Verification items for the finished model (mm, model axes). A direction names the side the tool comes from. Round coordinates to 2 decimals unless told otherwise and drop trailing zeros. Write each loop counter-clockwise with the first axis right and the second up, starting at its lowest first coordinate (ties: lowest second). Pieces come first, ordered by that corner, then holes. Notation, with made-up numbers: (-20.75, -30.75) -> (11.25, -30.75) arc R8 ccw to (11.25, -19.75) -> close; hole circle Ø6 at (39.25, 74). An arc over 180 degrees is marked (long way). Answer as a JSON object with one key per item and string values. Group by question number.
(1) Sectioned sample at B-B on z = 25.5. Record the cut outline in (x, y) (3 decimals).
(2) Sectioned sample at A-A on x = 57. Record the cut outline in (y, z) (3 decimals), and give its area (3 significant figures).
(3) Sectioned sample at C-C on z = -37.5. Record the cut outline in (x, y) (3 decimals).
(4) Sectioned sample at D-D on z = 15. Record the cut outline in (x, y) (3 decimals), and give its area (3 significant figures).
(5) Set-up check for faces 4 (the face through (-4, 20.955, -31)), 5 (the face through (-79.106, 21.878, 0.284)), 6 (the face through (89, 22.225, 1)), 7 (the face through (89, 13, -41.275)), 8 (the face through (5, 22.225, -29)): record each of +Z, -Z, +X, -X, +Y, -Y from which the full face is reachable in a straight line by a thin tool's end or side.
(6) Scan lines: L1, parallel to X at y = 15.5, z = -22 (3 decimals); L2, parallel to Z at x = -49, y = 14.5 (3 decimals); L3, parallel to X at y = 23, z = -12 (3 decimals). Record each from-to range of solid material in increasing order. Write a range as from..to.
(7) Draft check along X on faces 1 (the face through (66.675, 9, 14)), 2 (the face through (-82.55, 7, 1)), 3 (the face through (81, 16, -6.35)). Enter one of: released by +X, released by -X, zero draft, split by the parting line, or undercut.
(8) Gauge pin test, flat ends, axial feed: pin 1 Ø3 at (y, z) = (15, 8) entering from -X (3 decimals); pin 2 Ø1 at (x, z) = (24.5, 28.5) entering from +Y (3 decimals); pin 3 Ø0.7 at (x, z) = (78.5, -6.5) entering from -Y (3 decimals). Record the tip position at first contact, or that the pin passes through.
```python
from build123d import *

# Parameters (mm, degrees)
SKETCH1_W           = 165.1
SKETCH1_H           = 88.9
BOSS_EXTRUDE1_DEPTH = 25.4
SKETCH2_W           = 82.55
SKETCH2_H           = 19.05
BOSS_EXTRUDE2_DEPTH = 12.7
SKETCH5_W           = 151.13
SKETCH5_H           = 70.358
CUT_EXTRUDE3_DEPTH  = 3.175
SKETCH7_W           = 165.1
SKETCH7_H           = 88.9
CUT_EXTRUDE4_DEPTH  = 3.175
CUT_EXTRUDE5_DEPTH  = 29.21
SKETCH11_W          = 142.477455076
SKETCH11_H          = 82.55
CUT_EXTRUDE7_DEPTH  = 17.78
SKETCH15_W          = 137.668
SKETCH15_H          = 57.404
CUT_EXTRUDE8_DEPTH  = 6.35
SKETCH19_W          = 12.7
SKETCH19_H          = 24.13
CUT_EXTRUDE9_DEPTH  = 17.78
SKETCH22_W          = 19.304
SKETCH22_H          = 12.7
CUT_EXTRUDE11_DEPTH = 7.62
CUT_EXTRUDE11_DRAFT = 15
SKETCH24_W          = 28.575
SKETCH24_H          = 19.05
CUT_EXTRUDE12_DEPTH = 5.08
CUT_EXTRUDE14_DEPTH = 30.48


with BuildPart() as part:
    # Sketch1 → Boss-Extrude1 (new body)
    with BuildSketch(Plane(origin=(0, 0, 0), x_dir=(1, 0, 0), z_dir=(0, 1, 0))):
        Rectangle(SKETCH1_W, SKETCH1_H)
    extrude(amount=BOSS_EXTRUDE1_DEPTH)

    # Sketch2 → Boss-Extrude2 (add)
    with BuildSketch(Plane(origin=(82.55, 0, 0), x_dir=(0, 0, -1), z_dir=(1, 0, 0))):
        with Locations((0, 12.7)):
            Rectangle(SKETCH2_W, SKETCH2_H)
    extrude(amount=BOSS_EXTRUDE2_DEPTH)

    # Sketch5 → Cut-Extrude3 (cut)
    with BuildSketch(Plane(origin=(0, 25.4, 0), x_dir=(1, 0, 0), z_dir=(0, 1, 0))):
        Rectangle(SKETCH5_W, SKETCH5_H)
    extrude(amount=-CUT_EXTRUDE3_DEPTH, mode=Mode.SUBTRACT)

    # Sketch7 → Cut-Extrude4 (cut)
    with BuildSketch(Plane.XZ):
        Rectangle(SKETCH7_W, SKETCH7_H)
    extrude(amount=-CUT_EXTRUDE4_DEPTH, mode=Mode.SUBTRACT)

    # Sketch9 → Cut-Extrude5 (cut)
    with BuildSketch(Plane(origin=(95.25, 0, 0), x_dir=(0, 0, -1), z_dir=(1, 0, 0))):
        with BuildLine():
            Line((6.985, 4.445), (-6.985, 4.445))
            ThreePointArc((-6.985, 4.445), (-12.065, 9.525), (-6.985, 14.605))
            Line((-6.985, 14.605), (6.985, 14.605))
            ThreePointArc((6.985, 14.605), (12.065, 9.525), (6.985, 4.445))
        make_face()
    extrude(amount=-CUT_EXTRUDE5_DEPTH, mode=Mode.SUBTRACT)

    # Sketch11 → Cut-Extrude7 (cut)
    with BuildSketch(Plane(origin=(0, 3.175, 0), x_dir=(-1, 0, 0), z_dir=(0, -1, 0))):
        with Locations((4.563727538, 0)):
            Rectangle(SKETCH11_W, SKETCH11_H)
    extrude(amount=-CUT_EXTRUDE7_DEPTH, mode=Mode.SUBTRACT)

    # Sketch15 → Cut-Extrude8 (cut)
    with BuildSketch(Plane(origin=(0, 22.225, 0), x_dir=(1, 0, 0), z_dir=(0, 1, 0))):
        Rectangle(SKETCH15_W, SKETCH15_H)
    extrude(amount=-CUT_EXTRUDE8_DEPTH, mode=Mode.SUBTRACT)

    # Sketch19 → Cut-Extrude9 (cut)
    with BuildSketch(Plane(origin=(0, 3.175, 0), x_dir=(-1, 0, 0), z_dir=(0, -1, 0))):
        with Locations((-73.025, -29.21)):
            Rectangle(SKETCH19_W, SKETCH19_H)
        with Locations((-73.025, 29.21)):
            Rectangle(SKETCH19_W, SKETCH19_H)
    extrude(amount=-CUT_EXTRUDE9_DEPTH, mode=Mode.SUBTRACT)


with BuildPart() as cut_extrude11_tool:
    # Sketch22 → Cut-Extrude11 (with draft: the straight prism first)
    with BuildSketch(Plane.ZY.offset(82.55)):
        with Locations((0.44501799, 14.605)):
            Rectangle(SKETCH22_W, SKETCH22_H)
    extrude(amount=-CUT_EXTRUDE11_DEPTH)
    # Cut-Extrude11: the draft: its side faces are tilted about the plane it starts from
    cut_extrude11_sides = [cut_extrude11_tool.faces().sort_by_distance(p)[0] for p in [
        (-78.74, 14.605, 10.09701799),
        (-78.74, 20.955, 0.44501799),
        (-78.74, 14.605, -9.20698201),
        (-78.74, 8.255, 0.44501799),
    ]]
    draft(cut_extrude11_sides, Plane.ZY.offset(82.55), CUT_EXTRUDE11_DRAFT)


with BuildPart() as part_1:
    add(part.part)

    # Cut-Extrude11: cut by cut_extrude11_tool
    add(cut_extrude11_tool.part, mode=Mode.SUBTRACT)

    # Sketch24 → Cut-Extrude12 (cut)
    with BuildSketch(Plane.XZ.offset(-3.175)):
        with Locations((80.9625, 0)):
            Rectangle(SKETCH24_W, SKETCH24_H)
    extrude(amount=-CUT_EXTRUDE12_DEPTH, mode=Mode.SUBTRACT)

    # Sketch27 → Cut-Extrude14 (cut)
    with BuildSketch(Plane(origin=(95.25, 0, 0), x_dir=(0, 0, -1), z_dir=(1, 0, 0))):
        Polygon((-6.985, 14.605), (-4.445, 14.605), (-4.445, 15.621), (-2.54, 15.621), (-2.54, 18.161), (-6.35, 18.161), (-6.35, 15.621), align=None)
        Polygon((2.54, 18.161), (2.54, 15.621), (4.445, 15.621), (4.445, 14.605), (6.35, 14.605), (6.35, 15.621), (6.35, 18.161), align=None)
    extrude(amount=-CUT_EXTRUDE14_DEPTH, mode=Mode.SUBTRACT)


solid = part_1.part
```
Computed values:
{
 "1": {"outline": "(-82.55, 3.175) -> (-75.802, 3.175) -> (-75.802, 20.955) -> (-68.834, 20.955) -> (-68.834, 22.225) -> (-75.565, 22.225) -> (-75.565, 25.4) -> (-82.55, 25.4) -> close; (68.834, 20.955) -> (79.375, 20.955) -> (79.375, 3.175) -> (95.25, 3.175) -> (95.25, 22.225) -> (82.55, 22.225) -> (82.55, 25.4) -> (75.565, 25.4) -> (75.565, 22.225) -> (68.834, 22.225) -> close"},
 "2": {"outline": "(3.175, -44.45) -> (25.4, -44.45) -> (25.4, -35.179) -> (22.225, -35.179) -> (22.225, -28.702) -> (20.955, -28.702) -> (20.955, -41.275) -> (3.175, -41.275) -> close; (3.175, 41.275) -> (20.955, 41.275) -> (20.955, 28.702) -> (22.225, 28.702) -> (22.225, 35.179) -> (25.4, 35.179) -> (25.4, 44.45) -> (3.175, 44.45) -> close", "area": "212 mm2"},
 "3": {"outline": "(-82.55, 3.175) -> (-75.802, 3.175) -> (-75.802, 20.955) -> (79.375, 20.955) -> (79.375, 3.175) -> (95.25, 3.175) -> (95.25, 22.225) -> (82.55, 22.225) -> (82.55, 25.4) -> (-82.55, 25.4) -> close"},
 "4": {"outline": "(-82.55, 3.175) -> (-75.802, 3.175) -> (-75.802, 20.955) -> (-68.834, 20.955) -> (-68.834, 22.225) -> (-75.565, 22.225) -> (-75.565, 25.4) -> (-82.55, 25.4) -> close; (66.675, 3.175) -> (95.25, 3.175) -> (95.25, 22.225) -> (82.55, 22.225) -> (82.55, 25.4) -> (75.565, 25.4) -> (75.565, 22.225) -> (68.834, 22.225) -> (68.834, 15.875) -> (66.675, 15.875) -> close", "area": "712 mm2"},
 "5": {"face 4": "-Y", "face 5": "none", "face 6": "+Z, -Z, +X, +Y", "face 7": "-Z, +X, +Y, -Y", "face 8": "+Y"},
 "6": {"L1": "-82.55..-75.802, 79.375..95.25", "L2": "-44.45..-41.275, 41.275..44.45", "L3": "-82.55..-75.565, 75.565..82.55"},
 "7": {"face 1": "undercut", "face 2": "released by -X", "face 3": "zero draft"},
 "8": {"pin 1": "x = 66.675", "pin 2": "y = 22.225", "pin 3": "y = 14.605"}
}
